The model under review builds one solid part; all positions refer to its coordinate system, in mm. Give positions to 0.01 mm unless a question says otherwise; leave off trailing zeros. Loops run counter-clockwise (first coordinate to the right, second up) from the corner with the lowest first, then second, coordinate; pieces in that order, holes last. Notation, with made-up numbers: M 12,-2 L 37,-2 A22 cw 37,27 Z; hole C 43,-25.5 d8. An arc over 180 degrees is marked long. Put each result on its own line as item: value. Start each with the question number.
```python
from build123d import *

# Parameters (mm, degrees)
SKETCH3_W             = 35.921024484
SKETCH3_H             = 35.921024484
BOSS_EXTRUDE2_DEPTH   = 12.7
BOSS_EXTRUDE3_DEPTH   = 25.4
F_8_CLEARANCE_HOLE1_D = 4.9149
F_8_CLEARANCE_HOLE2_D = 4.9149
FILLET1_R             = 2.54


with BuildPart() as part:
    # Sketch3 → Boss-Extrude2 (new body)
    with BuildSketch(Plane(origin=(0, 0, 0), x_dir=(1, 0, 0), z_dir=(0, 1, 0))):
        with Locations((17.960512242, -17.960512242)):
            Rectangle(SKETCH3_W, SKETCH3_H)
    extrude(amount=BOSS_EXTRUDE2_DEPTH)

    # Sketch4 → Boss-Extrude3 (add, symmetric)
    with BuildSketch(Plane(origin=(0, 0, 0), x_dir=(0.7071067811865476, 0, 0.7071067811865475), z_dir=(-0.7071067811865475, 0, 0.7071067811865476))):
        Polygon((25.4, 12.7), (-50.8, 12.7), (-76.2, 12.7), (-76.2, 0), (0, 0), (25.4, 0), align=None)
    extrude(amount=BOSS_EXTRUDE3_DEPTH, both=True)

    # #8 Clearance Hole1 (through all)
    with Locations(Plane(origin=(0, 0, 0), x_dir=(-1, 0, 0), z_dir=(0, -1, 0))):
        with Locations((-29.571024484, -29.571024484), (-4.171024484, -4.171024484), (-29.571024484, -4.171024484), (-4.171024484, -29.571024484), (4.809231637, 4.809231637)):
            Hole(F_8_CLEARANCE_HOLE1_D / 2)

    # #8 Clearance Hole2 (through all)
    with Locations(Plane(origin=(0, 12.7, 0), x_dir=(1, 0, 0), z_dir=(0, 1, 0))):
        with Locations((-55.35429873, 29.95813442), (-29.95813442, 55.35429873)):
            Hole(F_8_CLEARANCE_HOLE2_D / 2)

    # Fillet1
    fillet1_edges = [part.edges().sort_by_distance(p)[0] for p in [
        (-35.921024484, 6.35, -71.842048969),
        (-71.842048969, 6.35, -35.921024484),
        (35.921024484, 6.35, 0),
        (35.921024484, 6.35, 35.921024484),
        (0, 6.35, 35.921024484),
    ]]
    fillet(fillet1_edges, radius=FILLET1_R)


solid = part.part
```
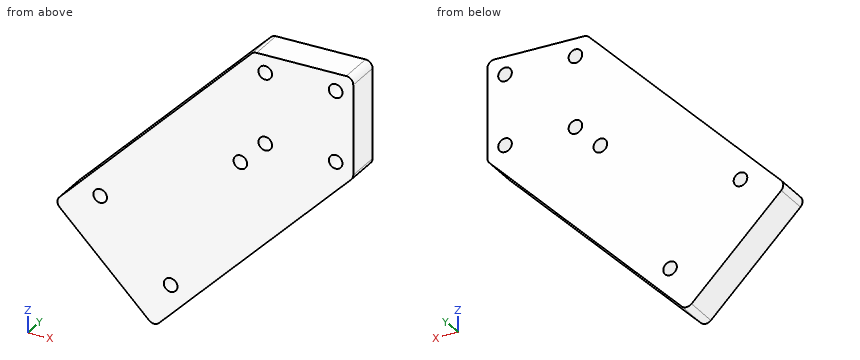
Item 1: Consider section C-C, the plane x = -49. Write out the cut boundary in (y, z), plus the area to 3 significant figures.
Item 2: Consider section B-B, the plane z = -50. Write out the cut boundary in (x, y), plus the area to 3 significant figures.
Item 3: To check wall thickness, follow L1, parallel to Z at x = 3, y = 9.5; L2, parallel to X at y = 9.5, z = -19; L3, parallel to X at y = 1, z = -42.5. State the ranges of each line that lie inside material, in increasing order. Write a range as [from, to].
Item 4: Consider section A-A, the plane y = 6. Write out the cut boundary in (x, z).
Item 5: Clearance check with flat-ended pins moving along their axes: pin 1 Ø1 at (y, z) = (1.5, -43.5) entering from +X; pin 2 Ø5 at (y, z) = (3, -3) entering from -X; pin 3 Ø5 at (y, z) = (5, 1.5) entering from -X. State where each tip first meets the part, or that it passes through.
Report:
1. outline: M 0,-58.76 L 12.7,-58.76 L 12.7,-13.08 L 0,-13.08 Z
1. area: 580 mm²
2. outline: M -57.76,0 L -14.08,0 L -14.08,12.7 L -57.76,12.7 Z
2. area: 555 mm²
3. L1: [-32.92, 2.01], [6.33, 27.41], [31.73, 35.92]
3. L2: [-54.92, 16.92]
3. L3: [-65.26, -6.58]
4. outline: M -70.05,-37.72 L -37.72,-70.05 A2.54 ccw -34.12,-70.05 L 35.18,-0.74 A2.54 ccw 35.92,1.05 L 35.92,33.38 A2.54 ccw 33.38,35.92 L 1.05,35.92 A2.54 ccw -0.74,35.18 L -70.05,-34.12 A2.54 ccw Z; hole C -55.35,-29.96 d4.91; hole C -29.96,-55.35 d4.91; hole C -4.81,-4.81 d4.91; hole C 4.17,4.17 d4.91; hole C 4.17,29.57 d4.91; hole C 29.57,4.17 d4.91; hole C 29.57,29.57 d4.91
5. pin 1: x = -7.08
5. pin 2: x = -41.42
5. pin 3: x = -36.92
